Answer from the drawing. Dimensions are ordinates in mm from the lowest x, y and z of the part. Coordinates: 2 decimals unless noted, no trailing zeros. Write each loop counter-clockwise with the first axis right and the second up, starting at its lowest first coordinate (ties: lowest second). Pieces come first, ordered by that corner, then holes.
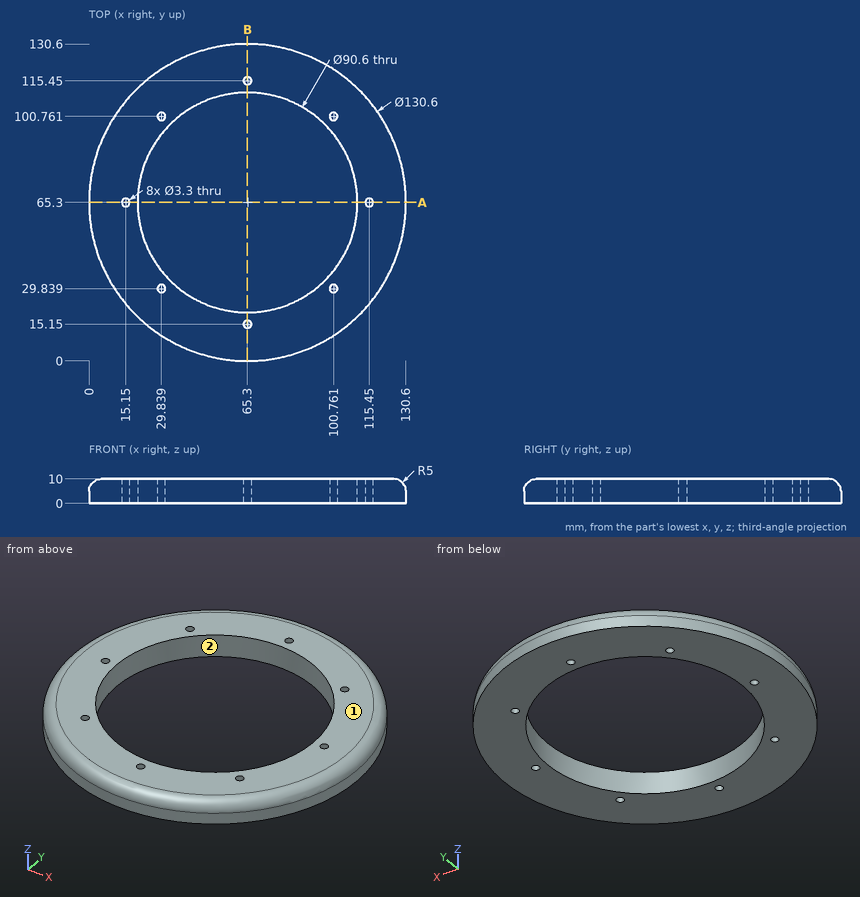
(1) For a pull along X with two mould halves and no side action, classify the marked faces 1 and 2 as pulls with the +X half, pulls with the -X half, needs draft (parallel to the pull), parting line crosses it, or undercut.
(2) Section B-B, the plane x = 65.3 is taken. State how many separate pieces and enclosed holes the cut face has, plus the area to 3 significant figures.
(3) Find the intervals of material crossed by probe 1 along Y at (x, z) = (65.3, 5.25); probe 2 along Y at (x, z) = (59, 4.25) (1 decimal); probe 3 along Y at (x, z) = (78, 2.75), in increasing order.
(4) Each of these flat-tipped pins is pushed along its axis until it touches: pin 1 (1 mm diameter, centred on x = 44.5, z = 5.5, fed in from -Y) (1 decimal); pin 2 (4 mm diameter, centred on y = 101, z = 6.5, fed in from +X); pin 3 (3 mm diameter, centred on x = 74, z = 7, fed in from +Y); pin 4 (3 mm diameter, centred on x = 65.3, y = 15.15, fed in from -Z). Where does it stop, or does it pass through?
(5) Section A-A, the plane y = 65.3 is taken. Write down the section's boundary in (x, z), plus the area to 3 significant figures.
Solution:
1. face 1: needs draft
1. face 2: undercut
2. separate pieces: 4
2. enclosed holes: 0
2. area: 323 mm2
3. probe 1: y = 0.01 to 13.5, 16.8 to 20, 110.6 to 113.8, 117.1 to 130.59
3. probe 2: y = 0.3 to 20.4, 110.2 to 130.3
3. probe 3: y = 1.25 to 21.82, 108.78 to 129.35
4. pin 1: stops at y = 3.3
4. pin 2: stops at x = 121.08
4. pin 3: stops at y = 130.07
4. pin 4: passes through
5. outline: (0, 0) - (13.5, 0) - (13.5, 10) - (5, 10) arc R5 ccw to (0, 5) - close; (16.8, 0) - (20, 0) - (20, 10) - (16.8, 10) - close; (110.6, 0) - (113.8, 0) - (113.8, 10) - (110.6, 10) - close; (117.1, 0) - (130.6, 0) - (130.6, 5) arc R5 ccw to (125.6, 10) - (117.1, 10) - close
5. area: 323 mm2
